Solid Edge part; units mm, degrees
sketch "Sketch1" plane through (0, 0, 0) normal (0, 0, 1) x (1, 0, 0)
  circle A0 centre (-6.75, 75.7107) radius 1.5
  circle A1 centre (6.75, 75.7107) radius 1.5
  line L0 (-9.75, 57.4107) -> (-21.25, 57.4107)
  line L1 (-21.25, 57.4107) -> (-21.25, 35.4107)
  line L2 (-21.25, 35.4107) -> (-9.75, 35.4107)
  line L3 (-9.75, 57.4107) -> (-9.75, 35.4107)
  circle A2 centre (17.7673, 40.9107) radius 1.5
  line L4 (50, -50) -> (50, 0)
  arc A3 (50, 0) -> (70.5719, -4.4281) centre (50, -50) cw
  arc A4 (70.5719, -4.4281) -> (49.5699, 50.4264) centre (0, 0) ccw
  arc A5 (-49.5699, 50.4264) -> (49.5699, 50.4264) centre (0, 24.5274) cw
  arc A6 (-70.5719, -4.4281) -> (-49.5699, 50.4264) centre (0, 0) cw
  arc A7 (-50, 0) -> (-70.5719, -4.4281) centre (-50, -50) ccw
  line L5 (-50, 0) -> (-50, -50)
  arc A8 (-50, -50) -> (50, -50) centre (0, 0) ccw
  dimension "D1" = 21.25
  dimension "D2" = 21.25
extrude "Protrusion1" add sketch "Sketch1" along normal blind 3
sketch "Sketch2" plane through (0, 4.8723, 0) normal (0, 0, -1) x (0, 1, 0)
  circle A0 centre (55.2883, -15.5) radius 1
  circle A1 centre (27.7883, -15.5) radius 1
  line L0 (25.0383, -6.5) -> (58.0383, -6.5)
  line L1 (58.0383, -6.5) -> (58.0383, -24.5)
  line L2 (58.0383, -24.5) -> (25.0383, -24.5)
  line L3 (25.0383, -24.5) -> (25.0383, -6.5)
extrude "ExtrudedProtrusion_2" add sketch "Sketch2" along normal blind 5
sketch "Sketch3" plane through (-15.5, 46.4107, 0) normal (0, 0, 1) x (1, 0, 0)
  line L0 (-5.75, 11) -> (5.75, 11)
  line L1 (5.75, 11) -> (5.75, -11)
  line L2 (5.75, -11) -> (-5.75, -11)
  line L3 (-5.75, -11) -> (-5.75, 10.8886)
extrude "Cutout1" cut sketch "Sketch3" against normal blind 126.1563 material side at (-15.5, 57.3607, 0)
sketch "Sketch4" plane through (0, 4.8723, 3) normal (0, 0, 1) x (0, 1, 0)
  circle A0 centre (-65.2277, 0) radius 1.5
  circle A1 centre (6.4136, 60.2859) radius 1.5
  circle A2 centre (6.4136, -60.2859) radius 1.5
extrude "ExtrudedProtrusion_3" add sketch "Sketch4" along normal blind 3
sketch "Sketch5" plane through (0, 4.8723, 0) normal (0, 0, -1) x (0, -1, 0)
  circle A0 centre (-6.4136, 60.2859) radius 1.5
  circle A1 centre (-6.4136, -60.2859) radius 1.5
extrude "ExtrudedCutout_3" cut sketch "Sketch5" against normal blind 1394.131
sketch "Sketch6" plane through (0, 4.8723, 0) normal (0, 0, -1) x (0, -1, 0)
  circle A0 centre (65.2277, 0) radius 1.5
extrude "ExtrudedCutout_4" cut sketch "Sketch6" against normal blind 239.0862
sketch "Sketch7" plane through (0, 4.8723, 3) normal (0, 0, 1) x (0, -1, 0)
  circle A0 centre (-55.2883, -15.5) radius 1
  circle A1 centre (-27.7883, -15.5) radius 1
extrude "ExtrudedCutout_5" cut sketch "Sketch7" against normal blind 54.4855
sketch "Sketch8" plane through (0, 4.8723, 3) normal (0, 0, 1) x (0, -1, 0)
  circle A0 centre (-19.655, 0) radius 55.928
extrude "ExtrudedProtrusion_4" add sketch "Sketch8" against normal blind 3
sketch "Sketch9" plane through (-15.5, 46.4107, -5) normal (0, 0, -1) x (-1, 0, 0)
  line L0 (-9, 16.5) -> (9, 16.5)
  line L1 (9, 16.5) -> (9, -16.5)
  line L2 (9, -16.5) -> (-9, -16.5)
  line L3 (-9, -16.5) -> (-9, 16.5)
  line L4 (-5.75, 11) -> (5.75, 11)
  line L5 (5.75, 11) -> (5.75, -11)
  line L6 (5.75, -11) -> (-5.75, -11)
  line L7 (-5.75, -11) -> (-5.75, 11)
extrude "ExtrudedCutout_6" cut sketch "Sketch9" against normal blind 5
sketch "Sketch10" plane through (0, 4.8723, 3) normal (0, 0, 1) x (0, -1, 0)
  line L0 (-13.0636, -10) -> (-13.0636, 10)
  line L1 (-13.0636, 10) -> (-33.2136, 10)
  line L2 (-33.2136, 10) -> (-53.3636, 10)
  line L3 (-53.3636, 10) -> (-53.3636, -10)
  line L4 (-53.3636, -10) -> (-33.2136, -10)
  line L5 (-33.2136, -10) -> (-13.0636, -10)
  circle A0 centre (-56.6886, -5.0517) radius 2.5
  circle A1 centre (-56.6886, 5) radius 2.5
  circle A2 centre (-9.7386, -5) radius 2.5
  circle A3 centre (-9.7386, 5) radius 2.5
extrude "ExtrudedProtrusion_5" add sketch "Sketch10" against normal blind 77.7502
sketch "Sketch11" plane through (0, 38.0859, -74.7502) normal (0, 0, -1) x (-1, 0, 0)
  line L0 (-10, 20.15) -> (10, 20.15)
  line L1 (10, 20.15) -> (10, -20.15)
  line L2 (10, -20.15) -> (-10, -20.15)
  line L3 (-10, -20.15) -> (-10, 20.15)
  circle A0 centre (-5, 23.475) radius 2.5
  circle A1 centre (5.0517, 23.475) radius 2.5
  circle A2 centre (5, -23.475) radius 2.5
  circle A3 centre (-5, -23.475) radius 2.5
extrude "ExtrudedCutout_7" cut sketch "Sketch11" against normal blind 2727.0102
sketch "Sketch12" plane through (0, 4.8723, 3) normal (0, 0, 1) x (0, -1, 0)
  line L0 (-53.3636, -10) -> (-60.0136, -10)
  line L1 (-60.0136, -10) -> (-60.0136, 10)
  line L2 (-60.0136, 10) -> (-53.3636, 10)
  line L3 (-53.3636, -10) -> (-53.3636, 10)
  line L4 (-13.0636, 10) -> (-6.4136, 10)
  line L5 (-6.4136, 10) -> (-6.4136, -10)
  line L6 (-6.4136, -10) -> (-13.0636, -10)
  line L7 (-13.0636, 10) -> (-13.0636, -10)
extrude "ExtrudedProtrusion_6" add sketch "Sketch12" against normal blind 3
sketch "Sketch13" plane through (0, 4.8723, 3) normal (0, 0, 1) x (0, -1, 0)
  circle A0 centre (-57.5136, 5) radius 2.5
  circle A1 centre (-57.5136, -5) radius 2.5
  circle A2 centre (-8.9136, 5) radius 2.5
  circle A3 centre (-8.9136, -5) radius 2.5
extrude "ExtrudedCutout_8" cut sketch "Sketch13" against normal blind 3
Geometry: final body of the model. Coordinates: model frame, mm. A direction names the side the tool comes from. Give positions to 0.01 mm unless a question says otherwise; leave off trailing zeros. Order: outer loops, then holes, each group sorted by start corner. A loop starts at its lowest first (then second) coordinate and runs counter-clockwise, first axis right, second up. Notation, with made-up numbers: (-13.5, 63) -> (0.5, 63) arc R13 cw to (0.5, 83) -> close; hole circle Ø4 at (29.5, 82). An arc over 180 degrees is marked (long way). Answer as a JSON object with one key per item and string values.
Q1. First-contact query: pin 1 (1.5 mm diameter, centred on x = -16.5, z = 0.5, fed in from -Y); pin 2 (2 mm diameter, centred on x = -52, y = -35, fed in from -Z); pin 3 (0.9 mm diameter, centred on x = -4.5, z = 2, fed in from -Y); pin 4 (0.9 mm diameter, centred on y = 41.5, z = 1, fed in from -X). Flat tips, straight axial feed; report the tip coordinate or a pass-through.
Entries:
{"pin 1": "stops at y = -68.93", "pin 2": "passes through", "pin 3": "stops at y = -70.59", "pin 4": "stops at x = -57.58"}
Q2. Section B-B (x = -5). Output: boundary loops of the cut face in (y, z), plus the area to 3 significant figures.
Entries:
{"outline": "(-70.53, 0) -> (11.29, 0) -> (11.29, 3) -> (-70.53, 3) -> close; (16.29, 0) -> (17.94, 0) -> (17.94, 3) -> (16.29, 3) -> close; (58.24, 0) -> (59.89, 0) -> (59.89, 3) -> (58.24, 3) -> close; (64.89, 0) -> (80.23, 0) -> (80.23, 3) -> (64.89, 3) -> close", "area": "301 mm^2"}
Q3. Section D-D (x = 37). Output: boundary loops of the cut face in (y, z), plus the area to 3 significant figures.
Entries:
{"outline": "(-60.26, 0) -> (66.47, 0) -> (66.47, 3) -> (-60.26, 3) -> close", "area": "380 mm^2"}
Q4. Section C-C (y = -26). Output: boundary loops of the cut face in (x, z), plus the area to 3 significant figures.
Entries:
{"outline": "(-50, 0) -> (50, 0) -> (50, 3) -> (-50, 3) -> close", "area": "300 mm^2"}
Q5. Section A-A (z = 1.25). State how many separate pieces and enclosed holes the cut face has, plus the area to 3 significant figures.
Entries:
{"separate pieces": "1", "enclosed holes": "8", "area": "14,200 mm^2"}
Q6. Access query for faces 1 (the cylindrical face through (-60.79, -1.18, 1.48)), 2 (the cylindrical face through (-4.89, 64.883, 1.521)). Directions: +Z, -Z, +X, -X, +Y, -Y. A direction counts if a zero-diameter tool reaches every point of the face in a straight line with its end or side. Return the directions, or none.
Entries:
{"face 1": "+Z, -Z, -Y", "face 2": "+Z, -Z"}
Q7. Material intervals for probe 1 along Y at (x, z) = (0, 0.9); probe 2 along X at (y, z) = (12, 1.2) (3 decimals); probe 3 along Y at (x, z) = (-6, 2.3), sorted ascending.
Entries:
{"probe 1": "y = -70.71 to -61.86, -58.86 to 17.94, 58.24 to 80.46", "probe 2": "x = -69.685 to -61.605, -58.967 to -6.749, -3.251 to 3.251, 6.749 to 58.967, 61.605 to 69.685", "probe 3": "y = -70.46 to 11.49, 16.08 to 17.94, 58.24 to 60.09, 64.68 to 80.13"}
Q8. Draft query along Y for faces 3 (the flat face through (-1, 6, 0)), 4 (the cylindrical face through (5.11, 16.283, 1.521)), 5 (the cylindrical face through (-4.89, 16.283, 1.521)), 6 (the cylindrical face through (60.507, -1.116, 1.479)). Return one class per face: released by +Y, released by -Y, zero draft, split by the parting line, or undercut.
Entries:
{"face 3": "zero draft", "face 4": "undercut", "face 5": "undercut", "face 6": "released by -Y"}
